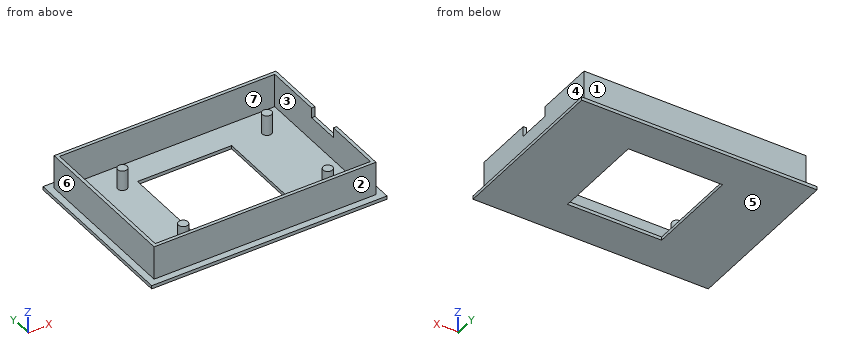
```python
from build123d import *

# Parameters (mm, degrees)
SKETCH005_W   = 70
SKETCH005_H   = 50
SKETCH005_W_2 = 28
SKETCH005_H_2 = 28
PAD_DEPTH     = 1
SKETCH006_R   = 1.4
PAD001_DEPTH  = 6
SKETCH007_W   = 66
SKETCH007_H   = 46
SKETCH007_W_2 = 64
SKETCH007_H_2 = 44
PAD002_DEPTH  = 10
SKETCH008_W   = 10
SKETCH008_H   = 3
POCKET_DEPTH  = 5


with BuildPart() as part:
    # Sketch005 → Pad (new body)
    with BuildSketch(Plane.XY):
        with Locations((35, 25)):
            Rectangle(SKETCH005_W, SKETCH005_H)
        with Locations((35, 25)):
            Rectangle(SKETCH005_W_2, SKETCH005_H_2, mode=Mode.SUBTRACT)
    extrude(amount=PAD_DEPTH)

    # Sketch006 → Pad001 (join)
    with BuildSketch(Plane.XY.offset(1)):
        with Locations((16.5, 39)):
            Circle(SKETCH006_R)
        with Locations((59.5, 39)):
            Circle(SKETCH006_R)
        with Locations((59.5, 11)):
            Circle(SKETCH006_R)
        with Locations((16.5, 11)):
            Circle(SKETCH006_R)
    extrude(amount=PAD001_DEPTH)

    # Sketch007 → Pad002 (join)
    with BuildSketch(Plane.XY.offset(1)):
        with Locations((35, 25)):
            Rectangle(SKETCH007_W, SKETCH007_H)
        with Locations((35, 25)):
            Rectangle(SKETCH007_W_2, SKETCH007_H_2, mode=Mode.SUBTRACT)
    extrude(amount=PAD002_DEPTH)

    # Sketch008 (on Face13 of Pad002) → Pocket (cut)
    with BuildSketch(Plane.YZ.offset(68)):
        with Locations((25, 9.5)):
            Rectangle(SKETCH008_W, SKETCH008_H)
    extrude(amount=-POCKET_DEPTH, mode=Mode.SUBTRACT)


solid = part.part
```
CAD build for the part. Positions are in the model's coordinates, mm. Face numbers are marked on the shaded views. A direction names the side the tool comes from. Give positions to 0.01 mm unless a question says otherwise; leave off trailing zeros. Order: outer loops, then holes, each group sorted by start corner. A loop starts at its lowest first (then second) coordinate and runs counter-clockwise, first axis right, second up. Notation, with made-up numbers: M 49,-9.75 L 82,-9.75 A4 ccw 82,-3.75 Z; hole C -34.75,11 d1. An arc over 180 degrees is marked long. Put each result on its own line as item: value. Start each with the question number.
(1) Saw through at B-B, the plane x = 59.5. Write the cut outline in (y, z).
(2) Drill centre lines: line 1 along X through (y, z) = (28, 5.75); line 2 along Y through (x, z) = (29, 10.75); line 3 along Z through (x, y) = (20, 14.5). Where is each one in solid material? Low to high.
(3) Which spindle directions (+Z, -Z, +X, -X, +Y, -Y) get a long thin tool onto all of the face, cutting with end or side? Do the marked faces 5, 6 and 7. Say none if no direction does.
(4) Flat gauge pins, fed straight in: pin 1 Ø3 at (x, z) = (14, 9) entering from +Y; pin 2 Ø1.1 at (x, y) = (67.5, 25) entering from +Z; pin 3 Ø4 at (y, z) = (37.5, 7) entering from +X. Where does each tip first touch, or does it go through?
(5) Saw through at A-A, the plane z = 3.5. Write the cut outline in (x, y), then the cut area to 3 significant figures.
(6) Saw through at C-C, the plane x = 30.5. Write the cut outline in (y, z).
(7) Mould opens along Y. For the marked faces 1, 2, 3 and 4 say: +Y half, -Y half, draft (parallel to the pull), parting line (faces both ways), or undercut.
Check result:
1. outline: M 0,0 L 50,0 L 50,1 L 48,1 L 48,11 L 47,11 L 47,1 L 40.4,1 L 40.4,7 L 37.6,7 L 37.6,1 L 12.4,1 L 12.4,7 L 9.6,7 L 9.6,1 L 3,1 L 3,11 L 2,11 L 2,1 L 0,1 Z
2. line 1: x = 2 to 3, 67 to 68
2. line 2: y = 2 to 3, 47 to 48
2. line 3: z = 0 to 1
3. face 5: -Z, +X, -X, +Y, -Y
3. face 6: +Z, -X, +Y, -Y
3. face 7: +Z
4. pin 1: stops at y = 48
4. pin 2: stops at z = 8
4. pin 3: stops at x = 68
5. outline: M 2,2 L 68,2 L 68,48 L 2,48 Z; C 16.5,11 d2.8; C 16.5,39 d2.8; C 59.5,11 d2.8; C 59.5,39 d2.8; hole M 3,3 L 67,3 L 67,47 L 3,47 Z
5. area: 245 mm2
6. outline: M 0,0 L 11,0 L 11,1 L 3,1 L 3,11 L 2,11 L 2,1 L 0,1 Z; M 39,0 L 50,0 L 50,1 L 48,1 L 48,11 L 47,11 L 47,1 L 39,1 Z
7. face 1: +Y half
7. face 2: -Y half
7. face 3: undercut
7. face 4: draft
